Design review of the part shown in the three views and the two pictorial views. Dimensions are in mm from the part's minimum x, y and z. A direction names the side the tool comes from. Coordinates: 2 decimals unless noted, no trailing zeros. Write each loop counter-clockwise with the first axis right and the second up, starting at its lowest first coordinate (ties: lowest second). Pieces come first, ordered by that corner, then holes. Notation, with made-up numbers: (84.5, 42) -> (127.5, 42) arc R12 cw to (127.5, 49) -> close; hole circle Ø3 at (-33.75, -12). An arc over 180 degrees is marked (long way). Answer in a Markdown table with one row per item. Add a question column.
Item 1: Clearance check with flat-ended pins moving along their axes: P1, Ø7.5, axis at y = 16, z = 30, coming from the -X side; P2, Ø8, axis at x = 42, y = 17, coming from the +Z side; P3, Ø10.5, axis at x = 88, z = 29, coming from the -Y side. State where each tip first meets the part, or that it passes through.
Item 2: Take a section at B-B, the plane y = 65.5. Write out the cut boundary in (x, z), and give its area (4 significant figures).
Item 3: Take a section at A-A, the plane z = 52.5. Write out the cut boundary in (x, y), and give its area (3 significant figures).
Item 4: Draft analysis for pull direction X (two halves, no side actions). For the marked faces 1, 2 and 3, state which applies: released by +X, released by -X, zero draft, split by the parting line, or undercut.
Item 5: Take a section at D-D, the plane x = 91. Write out the cut boundary in (y, z), and give its area (3 significant figures).
Item 6: For the marked faces 4, 5 and 6, list the 3-axis set-ups (+Z, -Z, +X, -X, +Y, -Y) from which the entire face can be reached by the end or side of a thin tool; tool diameter is ignored.
Item 7: To check wall thickness, follow line 1 (X direction, y = 23, z = 8.5); line 2 (X direction, y = 42.5, z = 54); line 3 (Y direction, x = 41.5, z = 25). State the ranges of each line that lie inside material, in increasing order.
Item 8: Take a section at C-C, the plane z = 19. Write out the cut boundary in (x, y).
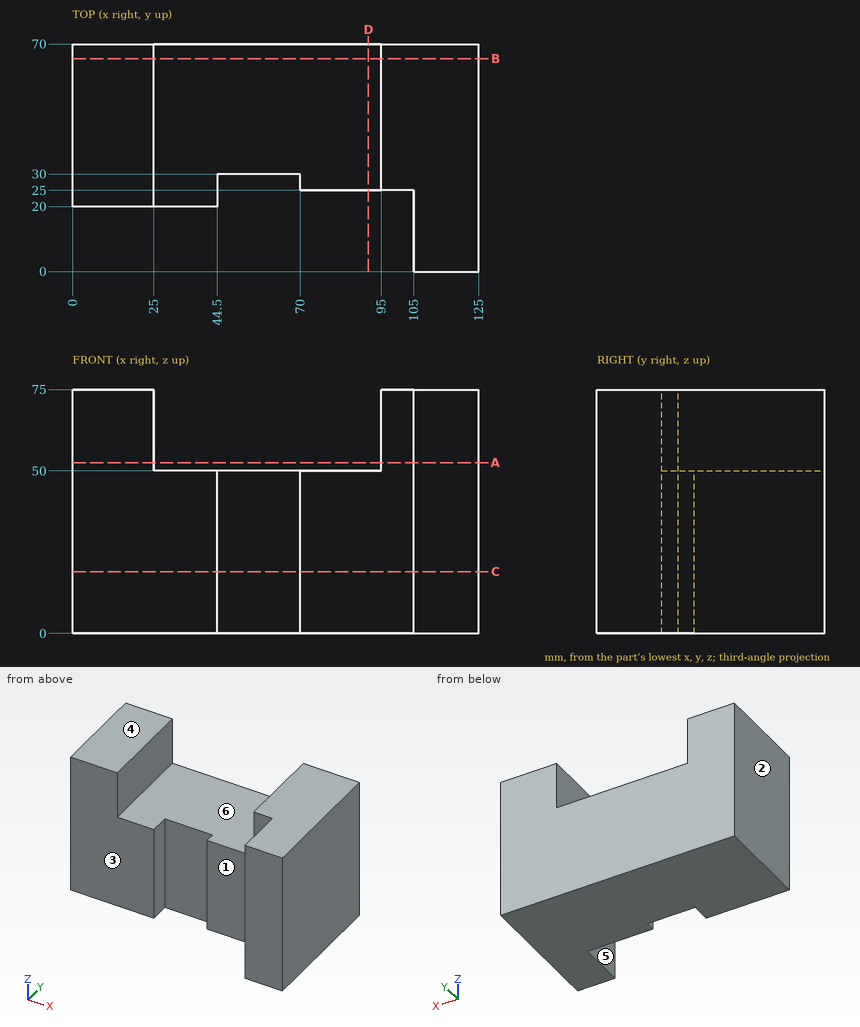
Answers:
| question | item | result |
|---|---|---|
| 1 | P1 | stops at x = 105 |
| 1 | P2 | stops at z = 50 |
| 1 | P3 | stops at y = 25 |
| 2 | outline | (0, 0) -> (125, 0) -> (125, 75) -> (95, 75) -> (95, 50) -> (25, 50) -> (25, 75) -> (0, 75) -> close |
| 2 | area | 7,625 mm^2 |
| 3 | outline | (0, 20) -> (25, 20) -> (25, 70) -> (0, 70) -> close; (95, 25) -> (105, 25) -> (105, 0) -> (125, 0) -> (125, 70) -> (95, 70) -> close |
| 3 | area | 3,100 mm^2 |
| 4 | face 1 | undercut |
| 4 | face 2 | released by -X |
| 4 | face 3 | zero draft |
| 5 | outline | (25, 0) -> (70, 0) -> (70, 50) -> (25, 50) -> close |
| 5 | area | 2,250 mm^2 |
| 6 | face 4 | +Z, +X, -X, +Y, -Y |
| 6 | face 5 | +Z, -Z, -Y |
| 6 | face 6 | +Z, +Y, -Y |
| 7 | line 1 | x = 0 to 44.5, 105 to 125 |
| 7 | line 2 | x = 0 to 25, 95 to 125 |
| 7 | line 3 | y = 20 to 70 |
| 8 | outline | (0, 20) -> (44.5, 20) -> (44.5, 30) -> (70, 30) -> (70, 25) -> (105, 25) -> (105, 0) -> (125, 0) -> (125, 70) -> (0, 70) -> close |
